```python
from build123d import *

# Parameters (mm, degrees)
SKETCH1_R           = 1.19
BOSS_EXTRUDE1_DEPTH = 1.64
SKETCH2_W           = 25.68
SKETCH2_H           = 2.47
BOSS_EXTRUDE2_DEPTH = 2.63
SKETCH3_W           = 0.65
SKETCH3_H           = 0.65
BOSS_EXTRUDE3_DEPTH = 5.64
CHAMFER1_SIZE       = 0.2


with BuildPart() as part:
    # Sketch1 → Boss-Extrude1 (new body)
    with BuildSketch(Plane(origin=(0, 0, 0), x_dir=(1, 0, 0), z_dir=(0, 1, 0))):
        with BuildLine():
            Line((-16.4125, 0), (16.4125, 0))
            ThreePointArc((16.4125, 0), (19, 2.5875), (16.4125, 5.175))
            Line((16.4125, 5.175), (13.975, 5.175))
            Line((13.975, 5.175), (13.975, 17.675))
            Line((13.975, 17.675), (16.4125, 17.675))
            ThreePointArc((16.4125, 17.675), (19, 20.2625), (16.4125, 22.85))
            Line((16.4125, 22.85), (-16.4125, 22.85))
            ThreePointArc((-16.4125, 22.85), (-19, 20.2625), (-16.4125, 17.675))
            Line((-16.4125, 17.675), (-13.975, 17.675))
            Line((-13.975, 17.675), (-13.975, 5.175))
            Line((-13.975, 5.175), (-16.4125, 5.175))
            ThreePointArc((-16.4125, 5.175), (-19, 2.5875), (-16.4125, 0))
        make_face()
        with Locations(Location((16.4125, 20.2625, 0), (0, 0, 270))):
            Circle(SKETCH1_R, mode=Mode.SUBTRACT)
        with Locations(Location((-16.4125, 20.2625, 0), (0, 0, 270))):
            Circle(SKETCH1_R, mode=Mode.SUBTRACT)
        with Locations(Location((-16.4125, 2.5875, 0), (0, 0, 270))):
            Circle(SKETCH1_R, mode=Mode.SUBTRACT)
        with Locations(Location((16.4125, 2.5875, 0), (0, 0, 270))):
            Circle(SKETCH1_R, mode=Mode.SUBTRACT)
    extrude(amount=BOSS_EXTRUDE1_DEPTH)

    # Sketch2 → Boss-Extrude2 (add)
    with BuildSketch(Plane(origin=(0, 1.64, 0), x_dir=(1, 0, 0), z_dir=(0, 1, 0))):
        with Locations((0, 2.215)):
            Rectangle(SKETCH2_W, SKETCH2_H)
    extrude(amount=BOSS_EXTRUDE2_DEPTH)

    # Sketch3 → Boss-Extrude3 (add)
    with BuildSketch(Plane(origin=(0, 4.27, 0), x_dir=(1, 0, 0), z_dir=(0, 1, 0))):
        with Locations((11.35, 2.215)):
            Rectangle(SKETCH3_W, SKETCH3_H)
        with Locations((8.827777778, 2.215)):
            Rectangle(SKETCH3_W, SKETCH3_H)
        with Locations((6.305555556, 2.215)):
            Rectangle(SKETCH3_W, SKETCH3_H)
        with Locations((3.783333333, 2.215)):
            Rectangle(SKETCH3_W, SKETCH3_H)
        with Locations((1.261111111, 2.215)):
            Rectangle(SKETCH3_W, SKETCH3_H)
        with Locations((-1.261111111, 2.215)):
            Rectangle(SKETCH3_W, SKETCH3_H)
        with Locations((-3.783333333, 2.215)):
            Rectangle(SKETCH3_W, SKETCH3_H)
        with Locations((-6.305555556, 2.215)):
            Rectangle(SKETCH3_W, SKETCH3_H)
        with Locations((-8.827777778, 2.215)):
            Rectangle(SKETCH3_W, SKETCH3_H)
        with Locations((-11.35, 2.215)):
            Rectangle(SKETCH3_W, SKETCH3_H)
    extrude(amount=BOSS_EXTRUDE3_DEPTH)

    # Chamfer1
    chamfer1_edges = [part.edges().sort_by_distance(p)[0] for p in [
        (3.783333333, 9.91, -1.89),
        (4.108333333, 9.91, -2.215),
        (1.261111111, 9.91, -2.54),
        (0.936111111, 9.91, -2.215),
        (1.261111111, 9.91, -1.89),
        (1.586111111, 9.91, -2.215),
        (-1.261111111, 9.91, -2.54),
        (-1.586111111, 9.91, -2.215),
        (-1.261111111, 9.91, -1.89),
        (-0.936111111, 9.91, -2.215),
        (-3.783333333, 9.91, -2.54),
        (-4.108333333, 9.91, -2.215),
        (-3.783333333, 9.91, -1.89),
        (-3.458333333, 9.91, -2.215),
        (-6.305555556, 9.91, -2.54),
        (-6.630555556, 9.91, -2.215),
        (-6.305555556, 9.91, -1.89),
        (-5.980555556, 9.91, -2.215),
        (-8.827777778, 9.91, -2.54),
        (-9.152777778, 9.91, -2.215),
        (-8.827777778, 9.91, -1.89),
        (-8.502777778, 9.91, -2.215),
        (-11.35, 9.91, -2.54),
        (-11.675, 9.91, -2.215),
        (-11.35, 9.91, -1.89),
        (-11.025, 9.91, -2.215),
        (11.675, 9.91, -2.215),
        (11.35, 9.91, -2.54),
        (11.025, 9.91, -2.215),
        (11.35, 9.91, -1.89),
        (8.827777778, 9.91, -2.54),
        (8.502777778, 9.91, -2.215),
        (8.827777778, 9.91, -1.89),
        (9.152777778, 9.91, -2.215),
        (6.305555556, 9.91, -2.54),
        (5.980555556, 9.91, -2.215),
        (6.305555556, 9.91, -1.89),
        (6.630555556, 9.91, -2.215),
        (3.783333333, 9.91, -2.54),
        (3.458333333, 9.91, -2.215),
    ]]
    chamfer(chamfer1_edges, length=CHAMFER1_SIZE)


solid = part.part
```
Could you check a few things on this model? Use its own coordinates, in mm. A direction names the side the tool comes from. Round coordinates to 2 decimals unless told otherwise and drop trailing zeros. Loops run counter-clockwise (first coordinate to the right, second up) from the corner with the lowest first, then second, coordinate; pieces in that order, holes last.
Q1. For P1, Ø5, axis at y = 2.5, z = -14, coming from the -X side (3 decimals); P2, Ø0.5, axis at y = 7.5, z = -2, coming from the +X side (3 decimals); P3, Ø0.7, axis at x = -4, y = 6.5, coming from the +Z side; P4, Ø2, axis at y = 4.5, z = -11.5, coming from the +X side, each with a flat end and sliding along its axis, tell me the tip position at first contact or that it passes through.
Q2. Thinking about a two-plate mould opening in X: for faces 1 (the flat face through (0, 3, -0.98)), 2 (the flat face through (-12.84, 3, -2)), 3 (the flat face through (0, 4.27, -2)), which applies, pulls with the +X half, pulls with the -X half, needs draft (parallel to the pull), parting line crosses it, or undercut?
Q3. I want a section at B-B (z = -19.5). Write out the boundary of the cut face in (x, y), and give its area (3 significant figures).
Q4. On a 3-axis mill with a long thin cutter (end or side, diameter ignored), from which of +Z, -Z, +X, -X, +Y, -Y can I reach the whole of each face in a straight line? I mean faces 4 (the flat face through (15, 1, -17.675)), 5 (the flat face through (-15, 1, -17.675)), 6 (the flat face through (0, 3, -3.45)), 7 (the flat face through (12.84, 3, -2)), 8 (the flat face through (0, 1, 0)). Say none if no direction works.
Q5. I want a section at A-A (x = 14.5). Write out the boundary of the cut face in (y, z) (3 decimals), and give its area (3 significant figures).
Q6. I want a section at C-C (y = 1.25). Give the number of separate pieces and of enclosed holes in the cut face, and give its area (3 significant figures).
Q7. I want a section at D-D (x = -10). Write out the boundary of the cut face in (y, z).
Q8. Please list where these lines run through material, in increasing order: L1, parallel to Y at x = -7, z = -12.5; L2, parallel to Z at x = 16, y = 1.5 (3 decimals); L3, parallel to Z at x = -3.5, y = 8.
Answer below:
1. P1: stops at x = -13.975
1. P2: stops at x = 11.675
1. P3: stops at z = -1.89
1. P4: passes through
2. face 1: needs draft
2. face 2: pulls with the -X half
2. face 3: undercut
3. outline: (-18.89, 0) - (-17.33, 0) - (-17.33, 1.64) - (-18.89, 1.64) - close; (-15.5, 0) - (15.5, 0) - (15.5, 1.64) - (-15.5, 1.64) - close; (17.33, 0) - (18.89, 0) - (18.89, 1.64) - (17.33, 1.64) - close
3. area: 55.9 mm2
4. face 4: +X, +Y, -Y
4. face 5: -X, +Y, -Y
4. face 6: -Z, +X, -X, +Y
4. face 7: +Z, -Z, +X, +Y
4. face 8: +Z, +X, -X, +Y, -Y
5. outline: (0, -22.85) - (1.64, -22.85) - (1.64, -17.675) - (0, -17.675) - close; (0, -5.175) - (1.64, -5.175) - (1.64, 0) - (0, 0) - close
5. area: 17.0 mm2
6. separate pieces: 1
6. enclosed holes: 4
6. area: 713 mm2
7. outline: (0, -22.85) - (1.64, -22.85) - (1.64, -3.45) - (4.27, -3.45) - (4.27, -0.98) - (1.64, -0.98) - (1.64, 0) - (0, 0) - close
8. L1: y = 0 to 1.64
8. L2: z = -22.85 to -21.379, -19.146 to -17.675, -5.175 to -3.704, -1.471 to 0
8. L3: z = -2.54 to -1.89
